Input: part model. Units: mm. Frame: model coordinates. Give positions to 0.01 mm unless a question says otherwise; leave off trailing zeros. Order: outer loops, then holes, each group sorted by start corner. A loop starts at its lowest first (then second) coordinate and runs counter-clockwise, first axis right, second up. Notation, with made-up numbers: (80, 4.25) - (84, 4.25) arc R10 ccw to (84, 14.25) - close; hole circle Ø6 at (-18.75, -15.5). An arc over 180 degrees is marked (long way). Use a Markdown table: item, result.
from build123d import *

# Parameters (mm, degrees)
EXTRUDE_1_DEPTH     = 55
SKETCH_2_R          = 2.1
CUT_EXTRUDE_1_DEPTH = 2.3
CHAMFER_1_SIZE      = 0.2
SKETCH_4_R          = 1.2
CUT_EXTRUDE_3_DEPTH = 56.167925464


with BuildPart() as part:
    # 草图1 → 凸台-拉伸1 (new body)
    with BuildSketch(Plane.XY):
        Polygon((-3.5, 0), (3.5, 0), (3.5, 2.4), (2.7, 3.2), (3.5, 4), (3.5, 4.8), (-3.5, 4.8), (-3.5, 4), (-2.7, 3.2), (-3.5, 2.4), align=None)
    extrude(amount=EXTRUDE_1_DEPTH)

    # 草图2 → 切除-拉伸1 (cut)
    with BuildSketch(Plane(origin=(0, 4.8, 0), x_dir=(1, 0, 0), z_dir=(0, 1, 0))):
        with Locations(Location((0, -5, 0), (0, 0, 180))):
            Circle(SKETCH_2_R)
        with Locations(Location((0, -20, 0), (0, 0, 180))):
            Circle(SKETCH_2_R)
        with Locations(Location((0, -35, 0), (0, 0, 180))):
            Circle(SKETCH_2_R)
        with Locations(Location((0, -50, 0), (0, 0, 180))):
            Circle(SKETCH_2_R)
    extrude(amount=-CUT_EXTRUDE_1_DEPTH, mode=Mode.SUBTRACT)

    # 倒角1
    chamfer_1_edges = [part.edges().sort_by_distance(p)[0] for p in [
        (-3.5, 4.8, 27.5),
        (3.5, 4.8, 27.5),
        (3.5, 0, 27.5),
        (-3.5, 0, 27.5),
    ]]
    chamfer(chamfer_1_edges, length=CHAMFER_1_SIZE)

    # 草图4 → 切除-拉伸3 (cut, through all)
    with BuildSketch(Plane(origin=(0, 2.5, 0), x_dir=(1, 0, 0), z_dir=(0, 1, 0))):
        with Locations(Location((0, -5, 0), (0, 0, 180))):
            Circle(SKETCH_4_R)
        with Locations(Location((0, -20, 0), (0, 0, 180))):
            Circle(SKETCH_4_R)
        with Locations(Location((0, -50, 0), (0, 0, 180))):
            Circle(SKETCH_4_R)
        with Locations(Location((0, -35, 0), (0, 0, 180))):
            Circle(SKETCH_4_R)
    extrude(amount=-CUT_EXTRUDE_3_DEPTH, mode=Mode.SUBTRACT)


solid = part.part
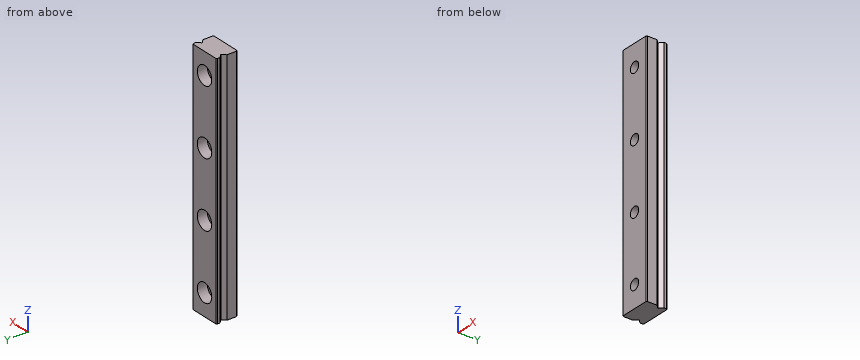
1. Pin query (flat end, axial travel): pin 1 (1.3 mm diameter, centred on x = 0.5, z = 49.5, fed in from +Y); pin 2 (2 mm diameter, centred on x = 0, z = 20, fed in from +Y); pin 3 (3 mm diameter, centred on x = 0, z = 50, fed in from -Y). Return the tip coordinate at first contact, or that it passes through.
Response:
| item | result |
|---|---|
| pin 1 | stops at y = 2.5 |
| pin 2 | passes through |
| pin 3 | stops at y = 0 |
2. Section query C-C (x = 0). State how many separate pieces and enclosed holes the cut face has, then the cut area to 3 significant figures.
Response:
| item | result |
|---|---|
| separate pieces | 5 |
| enclosed holes | 0 |
| area | 201 mm^2 |
3. Section query B-B (z = 20). Return loops of the section in (x, y).
Response:
| item | result |
|---|---|
| outline | (-3.5, 0.2) - (-3.3, 0) - (-1.2, 0) - (-1.2, 2.5) - (-2.1, 2.5) - (-2.1, 4.8) - (-3.3, 4.8) - (-3.5, 4.6) - (-3.5, 4) - (-2.7, 3.2) - (-3.5, 2.4) - close; (1.2, 0) - (3.3, 0) - (3.5, 0.2) - (3.5, 2.4) - (2.7, 3.2) - (3.5, 4) - (3.5, 4.6) - (3.3, 4.8) - (2.1, 4.8) - (2.1, 2.5) - (1.2, 2.5) - close |
4. Material intervals for line 1 along Z through (x, y) = (0, 3.7); line 2 along Z through (x, y) = (0, 1.25); line 3 along Y through (x, z) = (3.25, 32), sorted ascending.
Response:
| item | result |
|---|---|
| line 1 | z = 0 to 2.9, 7.1 to 17.9, 22.1 to 32.9, 37.1 to 47.9, 52.1 to 55 |
| line 2 | z = 0 to 3.8, 6.2 to 18.8, 21.2 to 33.8, 36.2 to 48.8, 51.2 to 55 |
| line 3 | y = 0 to 2.65, 3.75 to 4.8 |
5. Section query A-A (y = 0.8). Return loops of the section in (x, z), then the cut area to 3 significant figures.
Response:
| item | result |
|---|---|
| outline | (-3.5, 0) - (3.5, 0) - (3.5, 55) - (-3.5, 55) - close; hole circle Ø2.4 at (0, 5); hole circle Ø2.4 at (0, 20); hole circle Ø2.4 at (0, 35); hole circle Ø2.4 at (0, 50) |
| area | 367 mm^2 |
6. Section query D-D (z = 8). Return loops of the section in (x, y), then the cut area to 3 significant figures.
Response:
| item | result |
|---|---|
| outline | (-3.5, 0.2) - (-3.3, 0) - (3.3, 0) - (3.5, 0.2) - (3.5, 2.4) - (2.7, 3.2) - (3.5, 4) - (3.5, 4.6) - (3.3, 4.8) - (-3.3, 4.8) - (-3.5, 4.6) - (-3.5, 4) - (-2.7, 3.2) - (-3.5, 2.4) - close |
| area | 32.2 mm^2 |
